Could you check a few things on this model? Use its own coordinates, in mm. A direction names the side the tool comes from. Round coordinates to 2 decimals unless told otherwise and drop trailing zeros. Write each loop counter-clockwise with the first axis right and the second up, starting at its lowest first coordinate (ties: lowest second). Pieces come first, ordered by that corner, then holes. Notation, with made-up numbers: (-23.75, 89) -> (-3.75, 89) arc R7 cw to (-3.75, 94) -> close; hole circle Ø10 at (-5.5, 43). An arc over 180 degrees is marked (long way). Return JSON: item names as keys, results as strings.
from build123d import *

# Parameters (mm, degrees)
CROQUIS1_W              = 100
CROQUIS1_H              = 62
SALIENTE_EXTRUIR1_DEPTH = 35
CHAFL_N1_SIZE2          = 20.207259422
CHAFL_N1_SIZE           = 35
CROQUIS3_W              = 20
CROQUIS3_H              = 20
CORTAR_EXTRUIR1_DEPTH   = 38
CROQUIS4_W              = 20
CROQUIS4_H              = 20
CORTAR_EXTRUIR2_DEPTH   = 100
CROQUIS7_W              = 88
CROQUIS7_H              = 27
CORTAR_EXTRUIR5_DEPTH   = 30
CORTAR_EXTRUIR6_DEPTH   = 5
CROQUIS9_W              = 1.740341303
CROQUIS9_H              = 25
CROQUIS9_W_2            = 2.064222337
SALIENTE_EXTRUIR2_DEPTH = 25
CROQUIS10_W             = 100
CROQUIS10_H             = 10
SALIENTE_EXTRUIR3_DEPTH = 30
CROQUIS11_W             = 80.1
CROQUIS11_H             = 32
CORTAR_EXTRUIR7_DEPTH   = 5


with BuildPart() as part:
    # Croquis1 → Saliente-Extruir1 (new body)
    with BuildSketch(Plane(origin=(0, 0, 0), x_dir=(1, 0, 0), z_dir=(0, 1, 0))):
        with Locations((50, 31)):
            Rectangle(CROQUIS1_W, CROQUIS1_H)
    extrude(amount=SALIENTE_EXTRUIR1_DEPTH)

    # Chaflán1
    chafl_n1_edges = [part.edges().sort_by_distance(p)[0] for p in [
        (50, 35, 0),
    ]]
    chafl_n1_side = [part.faces().sort_by_distance(p)[0] for p in [
        (50, 34.595854812, 0),
    ]]
    chamfer(chafl_n1_edges, length=CHAFL_N1_SIZE - 0.0001, length2=CHAFL_N1_SIZE2 - 0.0001, reference=chafl_n1_side[0])  # a hair under: the kernel refuses the full size

    # Croquis3 → Cortar-Extruir1 (cut)
    with BuildSketch(Plane.XY):
        with Locations((50, 15)):
            Rectangle(CROQUIS3_W, CROQUIS3_H)
        with Locations((16, 15)):
            Rectangle(CROQUIS3_W, CROQUIS3_H)
        with Locations((84, 15)):
            Rectangle(CROQUIS3_W, CROQUIS3_H)
    extrude(amount=-CORTAR_EXTRUIR1_DEPTH, mode=Mode.SUBTRACT)

    # Croquis4 → Cortar-Extruir2 (cut)
    with BuildSketch(Plane.ZY):
        with Locations((-48, 15)):
            Rectangle(CROQUIS4_W, CROQUIS4_H)
    extrude(amount=-CORTAR_EXTRUIR2_DEPTH, mode=Mode.SUBTRACT)

    # Croquis7 → Cortar-Extruir5 (cut)
    with BuildSketch(Plane(origin=(0, 35, 0), x_dir=(1, 0, 0), z_dir=(0, 1, 0))):
        with Locations((50, 44.5)):
            Rectangle(CROQUIS7_W, CROQUIS7_H)
    extrude(amount=-CORTAR_EXTRUIR5_DEPTH, mode=Mode.SUBTRACT)

    # Croquis8 → Cortar-Extruir6 (cut)
    with BuildSketch(Plane(origin=(0, 35, 0), x_dir=(1, 0, 0), z_dir=(0, 1, 0))):
        Polygon((9, 31), (23, 31), (43, 31), (57, 31), (77, 31), (91, 31), (91, 23.207259422), (77, 23.207259422), (57, 23.207259422), (43, 23.207259422), (23, 23.207259422), (9, 23.207259422), align=None)
    extrude(amount=-CORTAR_EXTRUIR6_DEPTH, mode=Mode.SUBTRACT)

    # Croquis9 → Saliente-Extruir2 (add)
    with BuildSketch(Plane(origin=(0, 5, 0), x_dir=(1, 0, 0), z_dir=(0, 1, 0))):
        with Locations((19.129829349, 45.5)):
            Rectangle(CROQUIS9_W, CROQUIS9_H)
        with Locations((81.032111168, 45.5)):
            Rectangle(CROQUIS9_W_2, CROQUIS9_H)
    extrude(amount=SALIENTE_EXTRUIR2_DEPTH)

    # Croquis10 → Saliente-Extruir3 (add)
    with BuildSketch(Plane(origin=(0, 0, -62), x_dir=(-1, 0, 0), z_dir=(0, 0, -1))):
        with Locations((-50, 30)):
            Rectangle(CROQUIS10_W, CROQUIS10_H)
    extrude(amount=SALIENTE_EXTRUIR3_DEPTH)

    # Croquis11 → Cortar-Extruir7 (cut)
    with BuildSketch(Plane(origin=(0, 35, 0), x_dir=(1, 0, 0), z_dir=(0, 1, 0))):
        with Locations((50, 74)):
            Rectangle(CROQUIS11_W, CROQUIS11_H)
    extrude(amount=-CORTAR_EXTRUIR7_DEPTH, mode=Mode.SUBTRACT)


solid = part.part
1) For faces 1 (the face through (9, 33, -27)), 2 (the face through (97, 15, -38)), 3 (the face through (84, 25, -23)), which set-ups out of +Z, -Z, +X, -X, +Y, -Y let a thin tool reach every point of the face, with its end or its side?
Return value:
{"face 1": "+Y", "face 2": "+X", "face 3": "+Z"}
2) Will these pins go through, and if not, where does the flat tip stop? pin 1 Ø9 at (x, y) = (65, 14) entering from -Z; pin 2 Ø1.5 at (x, z) = (76.5, -67.5) entering from -Y; pin 3 Ø0.6 at (x, y) = (81.5, 13) entering from +Z.
Return value:
{"pin 1": "z = -62", "pin 2": "y = 25", "pin 3": "z = -33"}
3) Thinking about a two-plate mould opening in X: for faces 4 (the face through (3, 25, -48)), 5 (the face through (9.95, 33, -74)), 6 (the face through (94, 20, -30)), which applies, pulls with the +X half, pulls with the -X half, needs draft (parallel to the pull), parting line crosses it, or undercut?
Return value:
{"face 4": "needs draft", "face 5": "undercut", "face 6": "undercut"}
4) I want a section at C-C, the plane y = 11.5. Please give me the cut outline in (x, z), and give its area (3 significant figures).
Return value:
{"outline": "(0, -62) -> (100, -62) -> (100, -58) -> (82.06, -58) -> (82.06, -33) -> (80, -33) -> (80, -58) -> (20, -58) -> (20, -33) -> (18.26, -33) -> (18.26, -58) -> (0, -58) -> close; (0, -38) -> (6, -38) -> (6, -6.64) -> (0, -6.64) -> close; (26, -31) -> (40, -31) -> (40, -6.64) -> (26, -6.64) -> close; (60, -31) -> (74, -31) -> (74, -6.64) -> (60, -6.64) -> close; (94, -38) -> (100, -38) -> (100, -6.64) -> (94, -6.64) -> close", "area": "1,550 mm²"}
5) If I drill on probe 1 along X at (y, z) = (16, -10); probe 2 along X at (y, z) = (24, -51); probe 3 along Y at (x, z) = (57.5, -25), over which ranges is the centre line in solid material (lowest first)? Write a range as [from, to].
Return value:
{"probe 1": "[0, 6], [26, 40], [60, 74], [94, 100]", "probe 2": "[18.26, 20], [80, 82.06]", "probe 3": "[0, 5], [25, 30]"}
6) I want a section at B-B, the plane z = -44. Please give me the cut outline in (x, y).
Return value:
{"outline": "(0, 0) -> (100, 0) -> (100, 5) -> (82.06, 5) -> (82.06, 30) -> (80, 30) -> (80, 5) -> (20, 5) -> (20, 30) -> (18.26, 30) -> (18.26, 5) -> (0, 5) -> close; (0, 25) -> (6, 25) -> (6, 35) -> (0, 35) -> close; (94, 25) -> (100, 25) -> (100, 35) -> (94, 35) -> close"}
